from build123d import *

# Parameters (mm, degrees)
P_IDAT_VYSUNUT_M1_DEPTH = 30
P_IDAT_START            = -2
SKICA2_R                = 1.15
P_IDAT_VYSUNUT_M2_DEPTH = 3
P_IDAT_VYSUNUT_M3_DEPTH = 1


with BuildPart() as part:
    # Skica1 → Přidat vysunutím1 (new body)
    with BuildSketch(Plane(origin=(0, 0, 0), x_dir=(1, 0, 0), z_dir=(0, 1, 0))):
        Polygon((-5, 0), (5, 0), (5, 1.6), (4, 2.6), (4, 3), (5, 3), (5, 3.6), (6.2, 3.6), (6.2, -1), (-6.2, -1), (-6.2, 3.6), (-5, 3.6), (-5, 3), (-4, 3), (-4, 2.6), (-5, 1.6), align=None)
    p_idat_vysunut_m1 = extrude(amount=P_IDAT_VYSUNUT_M1_DEPTH)

    # Skica2 → Přidat vysunutím2 (add)
    with BuildSketch(Plane.XY.offset(P_IDAT_START)):
        with BuildLine():
            Line((-8.8, 13), (-8.5, 13))
            ThreePointArc((-8.5, 13), (-6.873654403, 12.326345597), (-6.2, 10.7))
            Line((-6.2, 10.7), (-6.2, 13))
            Line((-6.2, 13), (-6.2, 17))
            Line((-6.2, 17), (-6.2, 19.3))
            ThreePointArc((-6.2, 19.3), (-6.873654403, 17.673654403), (-8.5, 17))
            Line((-8.5, 17), (-8.8, 17))
            ThreePointArc((-8.8, 17), (-10.143502884, 16.443502884), (-10.7, 15.1))
            Line((-10.7, 15.1), (-10.7, 14.9))
            ThreePointArc((-10.7, 14.9), (-10.143502884, 13.556497116), (-8.8, 13))
        make_face()
        with Locations((-8.45, 15)):
            Circle(SKICA2_R, mode=Mode.SUBTRACT)
    p_idat_vysunut_m2 = extrude(amount=P_IDAT_VYSUNUT_M2_DEPTH)

    # Skica3 → Přidat vysunutím3 (add)
    with BuildSketch(Plane.XY.offset(1)):
        with BuildLine():
            Line((-6.2, 30), (6.2, 30))
            Line((6.2, 30), (6.2, 33))
            Line((6.2, 33), (5.959807907, 33))
            ThreePointArc((5.959807907, 33), (0.150662271, 32.3427273), (-5.364776224, 30.404140537))
            Line((-5.364776224, 30.404140537), (-6.2, 30))
        make_face()
    p_idat_vysunut_m3 = extrude(amount=-P_IDAT_VYSUNUT_M3_DEPTH)

    # Zrcadlit2: Přidat vysunutím1, Přidat vysunutím2, Přidat vysunutím3 across plane
    add(p_idat_vysunut_m1.mirror(Plane(origin=(6.2, 30, -3.6), x_dir=(0, 0, 1), z_dir=(-1, 0, 0))))
    add(p_idat_vysunut_m2.mirror(Plane(origin=(6.2, 30, -3.6), x_dir=(0, 0, 1), z_dir=(-1, 0, 0))))
    add(p_idat_vysunut_m3.mirror(Plane(origin=(6.2, 30, -3.6), x_dir=(0, 0, 1), z_dir=(-1, 0, 0))))


solid = part.part
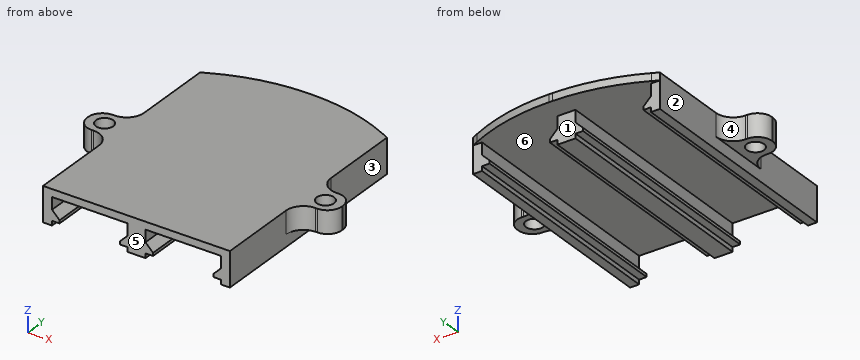
The listing builds one solid part. Answer for the finished solid, in the listing's coordinates (mm). Face numbers are marked on the shaded views. A direction names the side the tool comes from. Coordinates: 2 decimals unless noted, no trailing zeros. Loops run counter-clockwise (first coordinate to the right, second up) from the corner with the lowest first, then second, coordinate; pieces in that order, holes last. Notation, with made-up numbers: (55.5, 20) -> (105.5, 20) arc R17 ccw to (105.5, 52) -> close; hole circle Ø2 at (20, 36). An arc over 180 degrees is marked (long way). Answer in a Markdown table with one row per item. Add a question column.
1. Consider line 1 (X direction, y = 10.5, z = -3.25); line 2 (X direction, y = 3, z = -2.65); line 3 (Y direction, x = -8.45, z = 0.1). Determine where each line is inside the solid, lowest interval first. Write a range as [from, to].
2. Flat-ended cylindrical pins translate along their axes: P1, Ø2.5, axis at x = 17, z = -2, coming from the +Y side; P2, Ø2.5, axis at x = 20, y = 14, coming from the -Z side; P3, Ø0.5, axis at x = -4.5, y = 9, coming from the -Z side. Find the tip coordinate at first contact, or state that the pin passes through.
3. The part is cut by section A-A, the plane z = -0.85. Count the separate pieces of the cut face and the enclosed holes in it, then the cut area to 3 significant figures.
4. The part is cut by section B-B, the plane y = 26.5. Write down the section's boundary in (x, z), then the cut area to 3 significant figures.
5. For the marked faces 1, 2 and 3, determine the directions among +Z, -Z, +X, -X, +Y, -Y from which every point of the face is accessible in a straight line to the end or side of a thin tool.
6. Determine the mould class of the marked faces 4, 5 and 6 for opening direction X: +X half, -X half, draft (parallel to the pull), parting line (faces both ways), or undercut.
7. The part is cut by section D-D, the plane x = -1. Write down the section's boundary in (y, z).
8. The part is cut by section C-C, the plane x = 12. Write down the section's boundary in (y, z).
Answer below:
| question | item | result |
|---|---|---|
| 1 | line 1 | [-6.2, -5], [5, 7.4], [17.4, 18.6] |
| 1 | line 2 | [-6.2, -4], [4, 8.4], [16.4, 18.6] |
| 1 | line 3 | [13, 13.85], [16.15, 17] |
| 2 | P1 | y = 30 |
| 2 | P2 | z = -2 |
| 2 | P3 | z = -3 |
| 3 | separate pieces | 3 |
| 3 | enclosed holes | 2 |
| 3 | area | 173 mm2 |
| 4 | outline | (-6.2, -3.6) -> (-5, -3.6) -> (-5, -3) -> (-4, -3) -> (-4, -2.6) -> (-5, -1.6) -> (-5, 0) -> (5, 0) -> (5, -1.6) -> (4, -2.6) -> (4, -3) -> (5, -3) -> (5, -3.6) -> (7.4, -3.6) -> (7.4, -3) -> (8.4, -3) -> (8.4, -2.6) -> (7.4, -1.6) -> (7.4, 0) -> (17.4, 0) -> (17.4, -1.6) -> (16.4, -2.6) -> (16.4, -3) -> (17.4, -3) -> (17.4, -3.6) -> (18.6, -3.6) -> (18.6, 1) -> (-6.2, 1) -> close |
| 4 | area | 45.7 mm2 |
| 5 | face 1 | -Z, +X, -X, +Y |
| 5 | face 2 | -Z, -X |
| 5 | face 3 | -Z, +X |
| 6 | face 4 | -X half |
| 6 | face 5 | draft |
| 6 | face 6 | undercut |
| 7 | outline | (0, 0) -> (32.05, 0) -> (32.05, 1) -> (0, 1) -> close |
| 8 | outline | (0, 0) -> (32.4, 0) -> (32.4, 1) -> (0, 1) -> close |
